CAD build for the part. Positions are in the model's coordinates, mm. Round coordinates to 2 decimals unless told otherwise and drop trailing zeros. Write each loop counter-clockwise with the first axis right and the second up, starting at its lowest first coordinate (ties: lowest second). Pieces come first, ordered by that corner, then holes. Notation, with made-up numbers: (76.25, -38.75) -> (104.25, -38.75) arc R36 cw to (104.25, -3.75) -> close; hole circle Ø5 at (71, 36). An arc over 180 degrees is marked (long way). Put each result on its own line as item: value. Start each with the question number.
1. Saw through at B-B on z = 0. List the corners of the cut face in (x, y), and give its area (3 significant figures).
2. Saw through at C-C on x = 12.5. List the corners of the cut face in (y, z).
3. Saw through at A-A on y = 1.2. State how many separate pieces and enclosed holes the cut face has, and give its area (3 significant figures).
4. Drill centre lines: line 1 (X direction, y = 4.3, z = -2); line 2 (X direction, y = 0.7, z = -3.5); line 3 (X direction, y = 3.7, z = -6). Where is each one in solid material? Low to high. Write a range as from..to.
5. Flat gauge pins, fed straight in: P1, Ø2, axis at y = 3.5, z = 4, coming from the +X side; P2, Ø1, axis at y = 3.5, z = -9, coming from the -X side; P3, Ø2, axis at y = 3, z = -13.5, coming from the +X side. Where does each tip first touch, or does it go through?
6. Saw through at D-D on z = 13. List the corners of the cut face in (x, y).
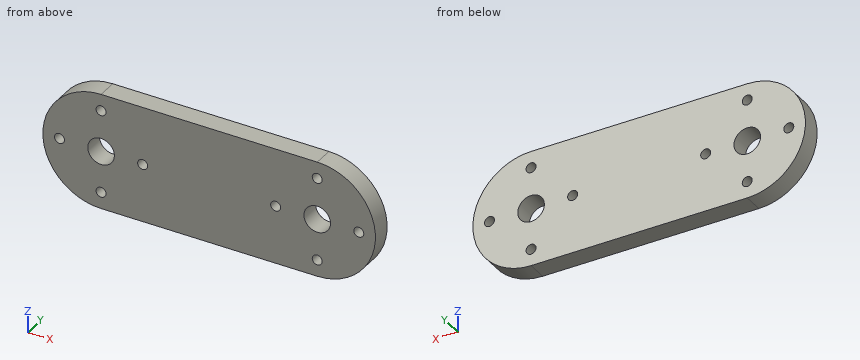
from build123d import *

# Parameters (mm, degrees)
SKETCH1_R           = 4
BOSS_EXTRUDE1_DEPTH = 6
SKETCH3_R           = 1.5
CUT_EXTRUDE1_DEPTH  = 19
SKETCH4_R           = 1.5
CUT_EXTRUDE2_DEPTH  = 19


with BuildPart() as part:
    # Sketch1 → Boss-Extrude1 (new body)
    with BuildSketch(Plane(origin=(0, 0, 0), x_dir=(1, 0, 0), z_dir=(0, 1, 0))):
        with BuildLine():
            Line((0, 17.5), (65, 17.5))
            ThreePointArc((65, 17.5), (82.5, 0), (65, -17.5))
            Line((65, -17.5), (0, -17.5))
            ThreePointArc((0, -17.5), (-17.5, 0), (0, 17.5))
        make_face()
        with Locations(Location((65, 0, 0), (0, 0, 270))):
            Circle(SKETCH1_R, mode=Mode.SUBTRACT)
        with Locations(Location((0, 0, 0), (0, 0, 270))):
            Circle(SKETCH1_R, mode=Mode.SUBTRACT)
    extrude(amount=BOSS_EXTRUDE1_DEPTH)

    # Sketch3 → Cut-Extrude1 (cut)
    with BuildSketch(Plane(origin=(0, 6, 0), x_dir=(1, 0, 0), z_dir=(0, 1, 0))):
        with Locations(Location((0, 12.5, 0), (0, 0, 270))):
            Circle(SKETCH3_R)
        with Locations(Location((12.5, 0, 0), (0, 0, 270))):
            Circle(SKETCH3_R)
        with Locations(Location((0, -12.5, 0), (0, 0, 270))):
            Circle(SKETCH3_R)
        with Locations(Location((-12.5, 0, 0), (0, 0, 270))):
            Circle(SKETCH3_R)
    extrude(amount=-CUT_EXTRUDE1_DEPTH, mode=Mode.SUBTRACT)

    # Sketch4 → Cut-Extrude2 (cut)
    with BuildSketch(Plane(origin=(0, 6, 0), x_dir=(1, 0, 0), z_dir=(0, 1, 0))):
        with Locations(Location((77.5, 0, 0), (0, 0, 270))):
            Circle(SKETCH4_R)
        with Locations(Location((65, -12.5, 0), (0, 0, 270))):
            Circle(SKETCH4_R)
        with Locations(Location((52.5, 0, 0), (0, 0, 270))):
            Circle(SKETCH4_R)
        with Locations(Location((65, 12.5, 0), (0, 0, 270))):
            Circle(SKETCH4_R)
    extrude(amount=-CUT_EXTRUDE2_DEPTH, mode=Mode.SUBTRACT)


solid = part.part
Return value:
1. outline: (-17.5, 0) -> (-14, 0) -> (-14, 6) -> (-17.5, 6) -> close; (-11, 0) -> (-4, 0) -> (-4, 6) -> (-11, 6) -> close; (4, 0) -> (11, 0) -> (11, 6) -> (4, 6) -> close; (14, 0) -> (51, 0) -> (51, 6) -> (14, 6) -> close; (54, 0) -> (61, 0) -> (61, 6) -> (54, 6) -> close; (69, 0) -> (76, 0) -> (76, 6) -> (69, 6) -> close; (79, 0) -> (82.5, 0) -> (82.5, 6) -> (79, 6) -> close
1. area: 432 mm^2
2. outline: (0, -17.5) -> (6, -17.5) -> (6, -1.5) -> (0, -1.5) -> close; (0, 1.5) -> (6, 1.5) -> (6, 17.5) -> (0, 17.5) -> close
3. separate pieces: 1
3. enclosed holes: 10
3. area: 3,080 mm^2
4. line 1: x = -17.39..-3.46, 3.46..61.54, 68.46..82.39
4. line 2: x = -17.15..-1.94, 1.94..63.06, 66.94..82.15
4. line 3: x = -16.44..81.44
5. P1: stops at x = 82.24
5. P2: stops at x = -15.3
5. P3: stops at x = 77.25
6. outline: (-11.72, 0) -> (-1.41, 0) -> (-1.41, 6) -> (-11.72, 6) -> close; (1.41, 0) -> (63.59, 0) -> (63.59, 6) -> (1.41, 6) -> close; (66.41, 0) -> (76.72, 0) -> (76.72, 6) -> (66.41, 6) -> close
